```python
from build123d import *

# Parameters (mm, degrees)
PAD_DEPTH               = 6.5
POCKET_DEPTH            = 5
PAD_MIRRORED_2_DEPTH    = 6.5
POCKET_MIRRORED_2_DEPTH = 5
FILLET_R                = 1


with BuildPart() as part:
    # Sketch → Pad (new body)
    with BuildSketch(Plane.XY):
        with BuildLine():
            ThreePointArc((9.3, 10.464703), (4.974644, 13.086364), (0, 14))
            Line((0, 4.5), (0, 14))
            ThreePointArc((4.5, 0), (3.181981, 3.181981), (0, 4.5))
            Line((4.5, 0), (9.3, 0))
            Line((9.3, 0), (9.3, 10.464703))
        make_face()
    pad = extrude(amount=PAD_DEPTH)

    # Sketch001 → Pocket (cut)
    with BuildSketch(Plane.XY.offset(6.5)):
        Polygon((7.621024, 0), (3.810512, 6.6), (-3.810512, 6.6), (-7.621024, 0), (-3.810512, -6.6), (3.810512, -6.6), align=None)
    pocket = extrude(amount=-POCKET_DEPTH, mode=Mode.SUBTRACT)

    # Sketch Mirrored 2 → Pad Mirrored 2 (add)
    with BuildSketch(Plane(origin=(0, 0, 0), x_dir=(-1, 0, 0), z_dir=(0, 0, -1))):
        with BuildLine():
            ThreePointArc((9.3, 10.464703), (4.974644, 13.086364), (0, 14))
            Line((0, 4.5), (0, 14))
            ThreePointArc((4.5, 0), (3.181981, 3.181981), (0, 4.5))
            Line((4.5, 0), (9.3, 0))
            Line((9.3, 0), (9.3, 10.464703))
        make_face()
    pad_mirrored_2 = extrude(amount=-PAD_MIRRORED_2_DEPTH)

    # Sketch001 Mirrored 2 → Pocket Mirrored 2 (cut)
    with BuildSketch(Plane(origin=(0, 0, 6.5), x_dir=(-1, 0, 0), z_dir=(0, 0, -1))):
        Polygon((7.621024, 0), (3.810512, 6.6), (-3.810512, 6.6), (-7.621024, 0), (-3.810512, -6.6), (3.810512, -6.6), align=None)
    pocket_mirrored_2 = extrude(amount=POCKET_MIRRORED_2_DEPTH, mode=Mode.SUBTRACT)

    # Mirrored001: Pad, Pocket, Pad Mirrored 2, Pocket Mirrored 2 across Sketch H_Axis
    add(pad.mirror(Plane.ZX))
    add(pocket.mirror(Plane.ZX), mode=Mode.SUBTRACT)
    add(pad_mirrored_2.mirror(Plane.ZX))
    add(pocket_mirrored_2.mirror(Plane.ZX), mode=Mode.SUBTRACT)

    # Fillet
    fillet_edges = [part.edges().sort_by_distance(p)[0] for p in [
        (-9.3, -5.232351, 6.5),
        (9.3, -5.232351, 6.5),
        (4.974644, -13.086364, 6.5),
        (4.974644, 13.086364, 6.5),
        (4.974644, -13.086364, 0),
        (9.3, -5.232351, 0),
        (-9.3, -5.232351, 0),
        (-4.974644, 13.086364, 0),
        (9.3, -10.464703, 3.25),
        (-9.3, -10.464703, 3.25),
        (-9.3, 10.464703, 3.25),
        (9.3, 10.464703, 3.25),
    ]]
    fillet(fillet_edges, radius=FILLET_R)


solid = part.part
```
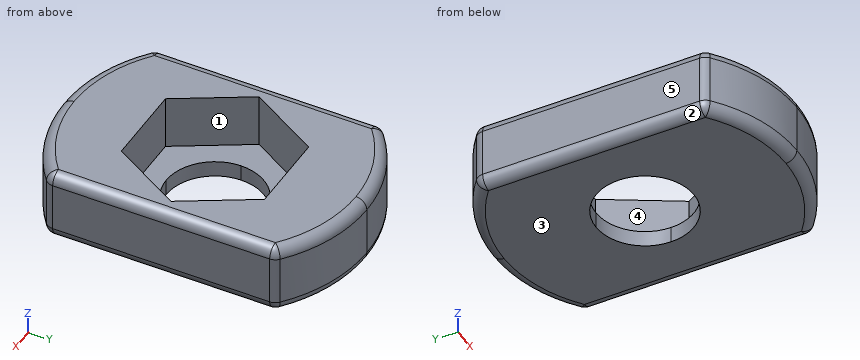
Could you check a few things on this model? Use its own coordinates, in mm. Face numbers are marked on the shaded views. A direction names the side the tool comes from. Give positions to 0.01 mm unless a question says otherwise; leave off trailing zeros. Write each loop counter-clockwise with the first axis right and the second up, starting at its lowest first coordinate (ties: lowest second). Pieces come first, ordered by that corner, then holes. Notation, with made-up numbers: (41, 66) -> (97, 66) arc R17 cw to (97, 91) -> close; hole circle Ø3 at (65, 62). An arc over 180 degrees is marked (long way). Write each question's results on one line, items separated by ' | '.
1. I want a section at B-B, the plane y = -1. Write out the boundary of the cut face in (x, z).
Check sheet entries:
outline: (-9.3, 1) arc R1 ccw to (-8.3, 0) -> (-4.39, 0) -> (-4.39, 1.5) -> (-7.04, 1.5) -> (-7.04, 6.5) -> (-8.3, 6.5) arc R1 ccw to (-9.3, 5.5) -> close; (4.39, 0) -> (8.3, 0) arc R1 ccw to (9.3, 1) -> (9.3, 5.5) arc R1 ccw to (8.3, 6.5) -> (7.04, 6.5) -> (7.04, 1.5) -> (4.39, 1.5) -> close
2. I need wall thicknesses on L1, parallel to Y at x = 2.5, z = 5; L2, parallel to X at y = -1.5, z = 5.5 (3 decimals); L3, parallel to Y at x = -6.5, z = 1.75. Which ranges of each line are inside material? Lowest first, please.
Check sheet entries:
L1: y = -13.77 to -6.6, 6.6 to 13.77 | L2: x = -9.3 to -6.755, 6.755 to 9.3 | L3: y = -12.4 to -1.94, 1.94 to 12.4
3. If we mould it in two halves opening along X, with no side actions, what happens to the marked faces 1, 2 and 3? For each: released by +X, released by -X, zero draft, split by the parting line, or undercut.
Check sheet entries:
face 1: undercut | face 2: released by -X | face 3: zero draft
4. I want a section at C-C, the plane y = -5.25. Write out the boundary of the cut face in (x, z), then the cut area to 3 significant figures.
Check sheet entries:
outline: (-9.3, 1) arc R1 ccw to (-8.3, 0) -> (8.3, 0) arc R1 ccw to (9.3, 1) -> (9.3, 5.5) arc R1 ccw to (8.3, 6.5) -> (4.59, 6.5) -> (4.59, 1.5) -> (-4.59, 1.5) -> (-4.59, 6.5) -> (-8.3, 6.5) arc R1 ccw to (-9.3, 5.5) -> close | area: 74.1 mm²
5. On a 3-axis mill with a long thin cutter (end or side, diameter ignored), from which of +Z, -Z, +X, -X, +Y, -Y can I reach the whole of each face in a straight line? I mean the marked faces 4 and 5. Say none if no direction works.
Check sheet entries:
face 4: +Z | face 5: +Z, -Z, -X, +Y, -Y
6. I want a section at D-D, the plane y = 2.25. Write out the boundary of the cut face in (x, z), then the cut area to 3 significant figures.
Check sheet entries:
outline: (-9.3, 1) arc R1 ccw to (-8.3, 0) -> (-3.9, 0) -> (-3.9, 1.5) -> (-6.32, 1.5) -> (-6.32, 6.5) -> (-8.3, 6.5) arc R1 ccw to (-9.3, 5.5) -> close; (3.9, 0) -> (8.3, 0) arc R1 ccw to (9.3, 1) -> (9.3, 5.5) arc R1 ccw to (8.3, 6.5) -> (6.32, 6.5) -> (6.32, 1.5) -> (3.9, 1.5) -> close | area: 45.1 mm²
7. I want a section at A-A, the plane z = 4.75. Write out the boundary of the cut face in (x, y).
Check sheet entries:
outline: (-9.3, -10.01) arc R1 ccw to (-8.94, -10.78) arc R14 ccw to (0, -14) arc R14 ccw to (8.94, -10.78) arc R1 ccw to (9.3, -10.01) -> (9.3, 10.01) arc R1 ccw to (8.94, 10.78) arc R14 ccw to (0, 14) arc R14 ccw to (-8.94, 10.78) arc R1 ccw to (-9.3, 10.01) -> close; hole (-7.62, 0) -> (-3.81, -6.6) -> (3.81, -6.6) -> (7.62, 0) -> (3.81, 6.6) -> (-3.81, 6.6) -> close
8. Will this pin go through, and if not, where does the flat tip stop? pin 1 Ø1.5 at (x, z) = (-1.5, 3) entering from +Y.
Check sheet entries:
pin 1: stops at y = 13.98
